Design review of the part built by this model. Coordinates are the model's own, in mm. Face numbers are marked on the shaded views. A direction names the side the tool comes from. Give positions to 0.01 mm unless a question says otherwise; leave off trailing zeros. Order: outer loops, then holes, each group sorted by start corner. A loop starts at its lowest first (then second) coordinate and runs counter-clockwise, first axis right, second up. Notation, with made-up numbers: (49.25, 26) -> (74.25, 26) arc R22 ccw to (74.25, 58) -> close; hole circle Ø11 at (-17, -30.75). An arc over 180 degrees is marked (long way). Use a Markdown table: item, result. Add a question column.
```python
from build123d import *

# Parameters (mm, degrees)
SKETCH1_R           = 67.5
BOSS_EXTRUDE1_DEPTH = 4
SKETCH2_R           = 7.5
CUT_EXTRUDE1_DEPTH  = 96.543183954
SKETCH3_R           = 10
CUT_EXTRUDE2_DEPTH  = 2.485754
CIRPATTERN1_START   = 1.514246464
CIRPATTERN1_DEPTH   = 2.485753536


# Read off the part's stored shape, not the designer's step: CirPattern1
with BuildPart() as part:
    # Sketch1 → Boss-Extrude1 (new body)
    with BuildSketch(Plane(origin=(0, 0, 0), x_dir=(1, 0, 0), z_dir=(0, 1, 0))):
        with Locations(Location((0, 0, 0), (0, 0, 270))):
            Circle(SKETCH1_R)
    extrude(amount=BOSS_EXTRUDE1_DEPTH)

    # Sketch2 → Cut-Extrude1 (cut, through all)
    with BuildSketch(Plane(origin=(0, 0, 0), x_dir=(1, 0, 0), z_dir=(0, 1, 0))):
        with Locations(Location((0, 0, 0), (0, 0, 270))):
            Circle(SKETCH2_R)
    extrude(amount=CUT_EXTRUDE1_DEPTH, mode=Mode.SUBTRACT)

    # Sketch3 → Cut-Extrude2 (cut)
    with BuildSketch(Plane(origin=(0, 4, 0), x_dir=(1, 0, 0), z_dir=(0, 1, 0))):
        with Locations(Location((-19.280397609, 0, 0), (0, 0, 270))):
            Circle(SKETCH3_R)
    extrude(amount=-CUT_EXTRUDE2_DEPTH, mode=Mode.SUBTRACT)

    # CirPattern1 outline → CirPattern1 (cut)
    with BuildSketch(Plane(origin=(0, 0, 0), x_dir=(1, 0, 0), z_dir=(0, 1, 0)).offset(CIRPATTERN1_START)):
        with BuildLine():
            ThreePointArc((4.233583399, -10.22077446), (0, -9.280397609), (-4.233583399, -10.22077446))
            ThreePointArc((-4.233583399, -10.22077446), (-6.562232082, -6.562232082), (-10.22077446, -4.233583399))
            ThreePointArc((-10.22077446, -4.233583399), (-15.453563285, -9.238795325), (-22.692923042, -9.399716494))
            ThreePointArc((-22.692923042, -9.399716494), (-20.704367705, -20.704367705), (-9.399716494, -22.692923042))
            ThreePointArc((-9.399716494, -22.692923042), (0, -29.280397609), (9.399716494, -22.692923042))
            ThreePointArc((9.399716494, -22.692923042), (20.704367705, -20.704367705), (22.692923042, -9.399716494))
            ThreePointArc((22.692923042, -9.399716494), (29.280397609, 0), (22.692923042, 9.399716494))
            ThreePointArc((22.692923042, 9.399716494), (20.704367705, 20.704367705), (9.399716494, 22.692923042))
            ThreePointArc((9.399716494, 22.692923042), (0, 29.280397609), (-9.399716494, 22.692923042))
            ThreePointArc((-9.399716494, 22.692923042), (-20.704367705, 20.704367705), (-22.692923042, 9.399716494))
            ThreePointArc((-22.692923042, 9.399716494), (-15.453563285, 9.238795325), (-10.22077446, 4.233583399))
            ThreePointArc((-10.22077446, 4.233583399), (-6.562232082, 6.562232082), (-4.233583399, 10.22077446))
            ThreePointArc((-4.233583399, 10.22077446), (0, 9.280397609), (4.233583399, 10.22077446))
            ThreePointArc((4.233583399, 10.22077446), (6.562232082, 6.562232082), (10.22077446, 4.233583399))
            ThreePointArc((10.22077446, 4.233583399), (9.280397609, 0), (10.22077446, -4.233583399))
            ThreePointArc((10.22077446, -4.233583399), (6.562232082, -6.562232082), (4.233583399, -10.22077446))
        make_face()
    extrude(amount=CIRPATTERN1_DEPTH, mode=Mode.SUBTRACT)


solid = part.part
```
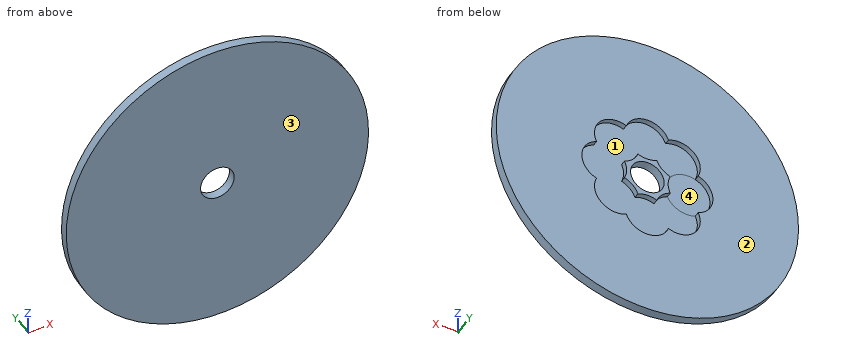
1) Insertion check: pin 1 (1.5 mm diameter, centred on x = -4.5, z = 9, fed in from -Y); pin 2 (18 mm diameter, centred on x = -19.28, z = 0, fed in from +Y); pin 3 (1 mm diameter, centred on x = -16.5, y = 1, fed in from +Z); pin 4 (13.5 mm diameter, centred on x = 0, z = 0, fed in from -Y). Each pin has a flat end and moves straight along its axis. Give the tip position at first contact, or say it passes through.
2) For L1, parallel to Z at x = 3.5, y = 2.15; L2, parallel to X at y = 2, z = -5; L3, parallel to Z at x = -2, y = 0.35, list the stretches that pass through material, from the lowest coordinate up. Write a range as [from, to].
3) Add section C-C (y = 3). Give the boundary of the cut face in (x, z).
4) Add section A-A (z = 0). Give the boundary of the cut face in (x, y), then the cut area to 3 significant figures.
5) Add section D-D (x = 15.5). Give the boundary of the cut face in (y, z).
6) Machinability: for the marked faces 3 and 4, which of the approach directions +Z, -Z, +X, -X, +Y, -Y give a long, thin tool a straight path to every point of the face, cutting with its end or side? Answer none if there is none.
7) The part is to be moulded in two halves that separate along Z. For the marked faces 1 and 2, say which applies: +Z half, -Z half, draft (parallel to the pull), parting line (faces both ways), or undercut.
8) Add section B-B (x = 0). Give the boundary of the cut face in (y, z).
Worked answers:
| question | item | result |
|---|---|---|
| 1 | pin 1 | y = 0 |
| 1 | pin 2 | y = 1.51 |
| 1 | pin 3 | z = 65.58 |
| 1 | pin 4 | through |
| 2 | L1 | [-67.41, -28.65], [-9.91, -6.63], [6.63, 9.91], [28.65, 67.41] |
| 2 | L2 | [-67.31, -27.94], [-8.59, -5.59], [5.59, 8.59], [27.94, 67.31] |
| 2 | L3 | [-67.47, -7.23], [7.23, 67.47] |
| 3 | outline | circle Ø135 at (0, 0); (-10.22, -4.23) arc R10 cw to (-4.23, -10.22) arc R10 cw to (4.23, -10.22) arc R10 cw to (10.22, -4.23) arc R10 cw to (10.22, 4.23) arc R10 cw to (4.23, 10.22) arc R10 cw to (-4.23, 10.22) arc R10 cw to (-10.22, 4.23) arc R10 cw to start; hole (-22.69, -9.4) arc R10 ccw to (-9.4, -22.69) arc R10 ccw to (9.4, -22.69) arc R10 ccw to (22.69, -9.4) arc R10 ccw to (22.69, 9.4) arc R10 ccw to (9.4, 22.69) arc R10 ccw to (-9.4, 22.69) arc R10 ccw to (-22.69, 9.4) arc R10 ccw to start; hole circle Ø15 at (0, 0) |
| 4 | outline | (-67.5, 0) -> (-7.5, 0) -> (-7.5, 4) -> (-9.28, 4) -> (-9.28, 1.51) -> (-29.28, 1.51) -> (-29.28, 4) -> (-67.5, 4) -> close; (7.5, 0) -> (67.5, 0) -> (67.5, 4) -> (29.28, 4) -> (29.28, 1.51) -> (9.28, 1.51) -> (9.28, 4) -> (7.5, 4) -> close |
| 4 | area | 381 mm^2 |
| 5 | outline | (0, -65.7) -> (4, -65.7) -> (4, -23.46) -> (1.51, -23.46) -> (1.51, 23.46) -> (4, 23.46) -> (4, 65.7) -> (0, 65.7) -> close |
| 6 | face 3 | +Z, -Z, +X, -X, -Y |
| 6 | face 4 | +Y |
| 7 | face 1 | undercut |
| 7 | face 2 | draft |
| 8 | outline | (0, -67.5) -> (4, -67.5) -> (4, -29.28) -> (1.51, -29.28) -> (1.51, -9.28) -> (4, -9.28) -> (4, -7.5) -> (0, -7.5) -> close; (0, 7.5) -> (4, 7.5) -> (4, 9.28) -> (1.51, 9.28) -> (1.51, 29.28) -> (4, 29.28) -> (4, 67.5) -> (0, 67.5) -> close |
